Part model, mm, in its own coordinate system. Face numbers are marked on the shaded views. A direction names the side the tool comes from. Round coordinates to 2 decimals unless told otherwise and drop trailing zeros. Loops run counter-clockwise (first coordinate to the right, second up) from the corner with the lowest first, then second, coordinate; pieces in that order, holes last. Notation, with made-up numbers: M 50,65.5 L 82,65.5 A14 cw 82,73.5 Z; hole C -30.5,-31 d7. An arc over 180 degrees is marked long. Put each result on its own line as item: value. Start each with the question number.
```python
from build123d import *

# Parameters (mm, degrees)
SKIZZE1_R                         = 2.5
SKIZZE1_R_2                       = 1
AUFSATZ_LINEAR_AUSTRAGEN1_DEPTH   = 17
AUFSATZ_LINEAR_AUSTRAGEN1_2_DEPTH = 17
AUFSATZ_LINEAR_AUSTRAGEN1_3_DEPTH = 17
AUFSATZ_LINEAR_AUSTRAGEN1_4_DEPTH = 17
SKIZZE1_3_W                       = 73.2
SKIZZE1_3_H                       = 69.3
SKIZZE1_3_W_2                     = 71.2
SKIZZE1_3_H_2                     = 67.3
AUFSATZ_LINEAR_AUSTRAGEN2_DEPTH   = 21
SKIZZE1_4_W                       = 71.2
SKIZZE1_4_H                       = 67.3
AUFSATZ_LINEAR_AUSTRAGEN3_DEPTH   = 19.5
SCHNITT_LINEAR_AUSTRAGEN1_DEPTH   = 2.1
SCHNITT_LINEAR_START              = -1
SCHNITT_LINEAR_AUSTRAGEN4_DEPTH   = 1.2
SCHNITT_LINEAR_START_2            = -66.9
SCHNITT_LINEAR_AUSTRAGEN6_DEPTH   = 1.4
AUFSATZ_LINEAR_AUSTRAGEN4_DEPTH   = 10
SCHNITT_LINEAR_AUSTRAGEN7_DEPTH   = 10
VERRUNDUNG1_R                     = 1
VERRUNDUNG2_R                     = 1


with BuildPart() as part:
    # Skizze1 → Aufsatz-Linear austragen1 (new body)
    with BuildSketch(Plane.XY):
        with Locations((63, 61.1)):
            Circle(SKIZZE1_R)
        with Locations((63, 61.1)):
            Circle(SKIZZE1_R_2, mode=Mode.SUBTRACT)
    extrude(amount=-AUFSATZ_LINEAR_AUSTRAGEN1_DEPTH)



with BuildPart() as body_2:
    # Skizze1 → Aufsatz-Linear austragen1 2 (new body)
    with BuildSketch(Plane.XY):
        with Locations((63, 3.1)):
            Circle(SKIZZE1_R)
        with Locations((63, 3.1)):
            Circle(SKIZZE1_R_2, mode=Mode.SUBTRACT)
    extrude(amount=-AUFSATZ_LINEAR_AUSTRAGEN1_2_DEPTH)


with BuildPart() as body_3:
    # Skizze1 → Aufsatz-Linear austragen1 3 (new body)
    with BuildSketch(Plane.XY):
        with Locations((8.5, 60.1)):
            Circle(SKIZZE1_R)
        with Locations((8.5, 60.1)):
            Circle(SKIZZE1_R_2, mode=Mode.SUBTRACT)
    extrude(amount=-AUFSATZ_LINEAR_AUSTRAGEN1_3_DEPTH)


with BuildPart() as body_4:
    # Skizze1 → Aufsatz-Linear austragen1 4 (new body)
    with BuildSketch(Plane.XY):
        with Locations((38, 3.1)):
            Circle(SKIZZE1_R)
        with Locations((38, 3.1)):
            Circle(SKIZZE1_R_2, mode=Mode.SUBTRACT)
    extrude(amount=-AUFSATZ_LINEAR_AUSTRAGEN1_4_DEPTH)


with BuildPart() as body_5:
    # Skizze1_3 → Aufsatz-Linear austragen2 (new body)
    with BuildSketch(Plane.XY):
        with Locations((34.5, 32.55)):
            Rectangle(SKIZZE1_3_W, SKIZZE1_3_H)
        with Locations((34.5, 32.55)):
            Rectangle(SKIZZE1_3_W_2, SKIZZE1_3_H_2, mode=Mode.SUBTRACT)
    extrude(amount=-AUFSATZ_LINEAR_AUSTRAGEN2_DEPTH)

    # Skizze1_4 → Aufsatz-Linear austragen3 (add)
    with BuildSketch(Plane.XY):
        with Locations((34.5, 32.55)):
            Rectangle(SKIZZE1_4_W, SKIZZE1_4_H)
        Polygon((36.5, 0), (0, 0), (0, 58.6), (0, 60.1), (0, 61.6), (0, 65.1), (7, 65.1), (8.5, 65.1), (10, 65.1), (61.5, 65.1), (63, 65.1), (64.5, 65.1), (69, 65.1), (69, 62.6), (69, 61.1), (69, 59.6), (69, 4.6), (69, 3.1), (69, 1.6), (69, 0), (64.5, 0), (63, 0), (61.5, 0), (39.5, 0), (38, 0), align=None, mode=Mode.SUBTRACT)
    extrude(amount=-AUFSATZ_LINEAR_AUSTRAGEN3_DEPTH)

    # Skizze2 → Schnitt-Linear austragen1 (cut)
    with BuildSketch(Plane(origin=(0, -2.1, 0), x_dir=(-1, 0, 0), z_dir=(0, -1, 0))):
        with BuildLine():
            ThreePointArc((-69.94600721, 21), (-34.5, 11.026332841), (0.94600721, 21))
            Line((0.94600721, 21), (-69.94600721, 21))
        make_face()
        with BuildLine():
            Line((-69.94600721, 21), (0.94600721, 21))
            ThreePointArc((0.94600721, 21), (24.786653318, 45.750756919), (33.473667159, 79))
            ThreePointArc((33.473667159, 79), (-67.749243081, 138.286653318), (-69.94600721, 21))
        make_face()
    extrude(amount=-SCHNITT_LINEAR_AUSTRAGEN1_DEPTH, mode=Mode.SUBTRACT)

    # Skizze2_6 → Schnitt-Linear austragen4 (cut)
    with BuildSketch(Plane(origin=(0, -2.1, 0), x_dir=(-1, 0, 0), z_dir=(0, -1, 0)).offset(SCHNITT_LINEAR_START)):
        with BuildLine():
            Line((0.94600721, 19.831196274), (0.94600721, 21))
            ThreePointArc((0.94600721, 21), (-34.5, 11.026332841), (-69.94600721, 21))
            Line((-69.94600721, 21), (-69.94600721, 19.831196274))
            ThreePointArc((-69.94600721, 19.831196274), (-34.5, 10.026332841), (0.94600721, 19.831196274))
        make_face()
    extrude(amount=-SCHNITT_LINEAR_AUSTRAGEN4_DEPTH, mode=Mode.SUBTRACT)

    # Skizze2_14 → Schnitt-Linear austragen6 (cut)
    with BuildSketch(Plane(origin=(0, -2.1, 0), x_dir=(-1, 0, 0), z_dir=(0, -1, 0)).offset(SCHNITT_LINEAR_START_2)):
        with BuildLine():
            Line((0.94600721, 19.831196274), (0.94600721, 21))
            ThreePointArc((0.94600721, 21), (-34.5, 11.026332841), (-69.94600721, 21))
            Line((-69.94600721, 21), (-69.94600721, 19.831196274))
            ThreePointArc((-69.94600721, 19.831196274), (-34.5, 10.026332841), (0.94600721, 19.831196274))
        make_face()
    extrude(amount=-SCHNITT_LINEAR_AUSTRAGEN6_DEPTH, mode=Mode.SUBTRACT)


with BuildPart() as part_1:
    add(part.part)

    add(body_2.part)  # Aufsatz-Linear austragen4 merges body 2

    add(body_3.part)  # Aufsatz-Linear austragen4 merges body 3

    add(body_4.part)  # Aufsatz-Linear austragen4 merges body 4

    add(body_5.part)  # Aufsatz-Linear austragen4 merges body 5
    # Skizze1_5 → Aufsatz-Linear austragen4 (add)
    with BuildSketch(Plane.XY):
        with BuildLine():
            Line((36.5, 1.1), (36.5, 0))
            Line((36.5, 0), (38, 0))
            Line((38, 0), (38, 0.6))
            ThreePointArc((38, 0.6), (37.209430585, 0.728291755), (36.5, 1.1))
        make_face()
        with BuildLine():
            Line((38, 0.6), (38, 0))
            Line((38, 0), (39.5, 0))
            Line((39.5, 0), (39.5, 1.1))
            ThreePointArc((39.5, 1.1), (38.790569415, 0.728291755), (38, 0.6))
        make_face()
        with BuildLine():
            Line((61.5, 1.1), (61.5, 0))
            Line((61.5, 0), (63, 0))
            Line((63, 0), (63, 0.6))
            ThreePointArc((63, 0.6), (62.209430585, 0.728291755), (61.5, 1.1))
        make_face()
        with BuildLine():
            Line((63, 0.6), (63, 0))
            Line((63, 0), (64.5, 0))
            Line((64.5, 0), (64.5, 1.1))
            ThreePointArc((64.5, 1.1), (63.790569415, 0.728291755), (63, 0.6))
        make_face()
        with BuildLine():
            Line((69, 4.6), (65, 4.6))
            ThreePointArc((65, 4.6), (65.371708245, 3.890569415), (65.5, 3.1))
            Line((65.5, 3.1), (69, 3.1))
            Line((69, 3.1), (69, 4.6))
        make_face()
        with BuildLine():
            Line((69, 3.1), (65.5, 3.1))
            ThreePointArc((65.5, 3.1), (65.371708245, 2.309430585), (65, 1.6))
            Line((65, 1.6), (69, 1.6))
            Line((69, 1.6), (69, 3.1))
        make_face()
        with BuildLine():
            Line((65.5, 61.1), (69, 61.1))
            Line((69, 61.1), (69, 62.6))
            Line((69, 62.6), (65, 62.6))
            ThreePointArc((65, 62.6), (65.371708245, 61.890569415), (65.5, 61.1))
        make_face()
        with BuildLine():
            Line((65, 59.6), (69, 59.6))
            Line((69, 59.6), (69, 61.1))
            Line((69, 61.1), (65.5, 61.1))
            ThreePointArc((65.5, 61.1), (65.371708245, 60.309430585), (65, 59.6))
        make_face()
        with BuildLine():
            Line((64.5, 65.1), (63, 65.1))
            Line((63, 65.1), (63, 63.6))
            ThreePointArc((63, 63.6), (63.790569415, 63.471708245), (64.5, 63.1))
            Line((64.5, 63.1), (64.5, 65.1))
        make_face()
        with BuildLine():
            Line((63, 65.1), (61.5, 65.1))
            Line((61.5, 65.1), (61.5, 63.1))
            ThreePointArc((61.5, 63.1), (62.209430585, 63.471708245), (63, 63.6))
            Line((63, 63.6), (63, 65.1))
        make_face()
        with BuildLine():
            Line((8.5, 65.1), (7, 65.1))
            Line((7, 65.1), (7, 62.1))
            ThreePointArc((7, 62.1), (7.709430585, 62.471708245), (8.5, 62.6))
            Line((8.5, 62.6), (8.5, 65.1))
        make_face()
        with BuildLine():
            ThreePointArc((8.5, 62.6), (9.290569415, 62.471708245), (10, 62.1))
            Line((10, 62.1), (10, 65.1))
            Line((10, 65.1), (8.5, 65.1))
            Line((8.5, 65.1), (8.5, 62.6))
        make_face()
        with BuildLine():
            Line((0, 61.6), (0, 60.1))
            Line((0, 60.1), (6, 60.1))
            ThreePointArc((6, 60.1), (6.128291755, 60.890569415), (6.5, 61.6))
            Line((6.5, 61.6), (0, 61.6))
        make_face()
        with BuildLine():
            Line((0, 60.1), (0, 58.6))
            Line((0, 58.6), (6.5, 58.6))
            ThreePointArc((6.5, 58.6), (6.128291755, 59.309430585), (6, 60.1))
            Line((6, 60.1), (0, 60.1))
        make_face()
    extrude(amount=-AUFSATZ_LINEAR_AUSTRAGEN4_DEPTH)

    # Skizze2_15 → Schnitt-Linear austragen7 (cut)
    with BuildSketch(Plane(origin=(0, -2.1, 0), x_dir=(-1, 0, 0), z_dir=(0, -1, 0)).offset(SCHNITT_LINEAR_START_2)):
        with BuildLine():
            ThreePointArc((-69.94600721, 21), (-34.5, 11.026332841), (0.94600721, 21))
            Line((0.94600721, 21), (-69.94600721, 21))
        make_face()
        with BuildLine():
            Line((-69.94600721, 21), (0.94600721, 21))
            ThreePointArc((0.94600721, 21), (24.786653318, 45.750756919), (33.473667159, 79))
            ThreePointArc((33.473667159, 79), (-67.749243081, 138.286653318), (-69.94600721, 21))
        make_face()
    extrude(amount=-SCHNITT_LINEAR_AUSTRAGEN7_DEPTH, mode=Mode.SUBTRACT)

    # Verrundung1
    verrundung1_edges = [part_1.edges().sort_by_distance(p)[0] for p in [
        (0, 65.1, -9.63732781),
        (69, 65.1, -9.63732781),
        (69, 0, -9.63732781),
        (0, 0, -9.63732781),
        (-2.1, -2.1, -10.5),
        (71.1, -2.1, -10.5),
        (71.1, 67.2, -10.5),
        (-2.1, 67.2, -10.5),
    ]]
    fillet(verrundung1_edges, radius=VERRUNDUNG1_R)

    # Verrundung2
    verrundung2_edges = [part_1.edges().sort_by_distance(p)[0] for p in [
        (70.1, 66.2, -20.25),
        (70.1, -1.1, -20.25),
        (-1.1, -1.1, -20.25),
        (-1.1, 66.2, -20.25),
    ]]
    fillet(verrundung2_edges, radius=VERRUNDUNG2_R)


solid = part_1.part
```
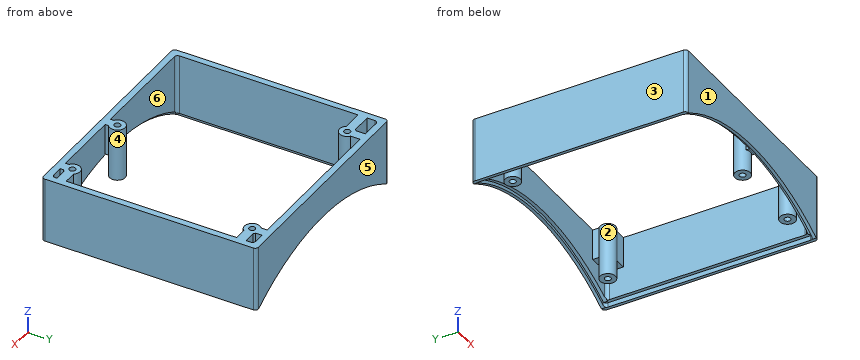
1. Cut at D-D, the plane x = 4.5. Give the cut face in (y, z).
2. Cut at A-A, the plane y = 3.1. Give the cut face in (x, z).
3. Cut at B-B, the plane x = 14.5. Give the cut face in (y, z), and give its area (3 significant figures).
4. Wall check: L1, parallel to Y at x = 63, z = -8.25; L2, parallel to Y at x = 63, z = -13.5; L3, parallel to X at y = 29, z = -9. Give the ranges that are in metal, low to high.
5. Which spindle directions (+Z, -Z, +X, -X, +Y, -Y) get a long thin tool onto all of the face, cutting with end or side? Do the marked faces 1 and 2. Say none if no direction does.
6. Mould opens along Y. For the marked faces 3, 4, 5 and 6 say: released by +Y, released by -Y, zero draft, split by the parting line, or undercut.
7. Cut at C-C, the plane y = 49. Give the cut face in (x, z).
8. Drop flat-ended pins along their axis: pin 1 (1.2 mm diameter, centred on x = 63.5, y = 0.5, fed in from -Z); pin 2 (1.5 mm diameter, centred on x = 67.5, y = 3, fed in from -Z). Give the stop position or say it passes through.
Results list:
1. outline: M -2.1,-18 L -1.1,-18 L -1.1,-16.89 L 0,-16.89 L 0,0 L -2.1,0 Z; M 58.6,-10 L 61.6,-10 L 61.6,0 L 58.6,0 Z; M 65.1,-16.89 L 66.2,-16.89 L 66.2,-18 L 67.2,-18 L 67.2,0 L 65.1,0 Z
2. outline: M -2.1,-21 L -1.1,-21 L -1.1,-19.5 L 0,-19.5 L 0,0 L -2.1,0 Z; M 35.5,-17 L 37,-17 L 37,0 L 35.5,0 Z; M 39,-17 L 40.5,-17 L 40.5,0 L 39,0 Z; M 60.5,-17 L 62,-17 L 62,0 L 60.5,0 Z; M 64,-17 L 65.5,-17 L 65.5,-10 L 69,-10 L 69,-19.5 L 70.1,-19.5 L 70.1,-21 L 71.1,-21 L 71.1,0 L 64,0 Z
3. outline: M -2.1,-14.04 L -1.1,-14.04 L -1.1,-12.99 L 0,-12.99 L 0,0 L -2.1,0 Z; M 65.1,-12.99 L 66.2,-12.99 L 66.2,-14.04 L 67.2,-14.04 L 67.2,0 L 65.1,0 Z
3. area: 56.6 mm^2
4. L1: y = -2.1 to 2.1, 4.1 to 5.6, 58.6 to 60.1, 62.1 to 67.2
4. L2: y = -2.1 to 0, 0.6 to 2.1, 4.1 to 5.6, 58.6 to 60.1, 62.1 to 63.6, 65.1 to 67.2
4. L3: x = -2.1 to 0, 69 to 71.1
5. face 1: +Z, -Z, +X, -X, -Y
5. face 2: -Z
6. face 3: zero draft
6. face 4: undercut
6. face 5: released by +Y
6. face 6: undercut
7. outline: M -2.1,-21 L -1.1,-21 L -1.1,-19.5 L 0,-19.5 L 0,0 L -2.1,0 Z; M 69,-19.5 L 70.1,-19.5 L 70.1,-21 L 71.1,-21 L 71.1,0 L 69,0 Z
8. pin 1: stops at z = -17
8. pin 2: stops at z = -10
